The listing builds one solid part. Answer for the finished solid, in the listing's coordinates (mm). A direction names the side the tool comes from. Round coordinates to 2 decimals unless told otherwise and drop trailing zeros. Loops run counter-clockwise (first coordinate to the right, second up) from the corner with the lowest first, then second, coordinate; pieces in that order, holes last. Notation, with made-up numbers: M 34,69.25 L 93,69.25 A26 ccw 93,97.25 Z; hole C 59,-21 d3. An arc over 180 degrees is marked long. Answer as a JSON object with one key per item and string values.
```python
from build123d import *

# Parameters (mm, degrees)
BOSS_EXTRUDE1_DEPTH = 20
SKETCH2_W           = 5
SKETCH2_H           = 20
BOSS_EXTRUDE2_DEPTH = 5
CUT_EXTRUDE1_DEPTH  = 5
SKETCH4_W           = 5
SKETCH4_H           = 5
BOSS_EXTRUDE3_DEPTH = 5
CUT_EXTRUDE2_DEPTH  = 5
BOSS_EXTRUDE4_DEPTH = 20
CUT_EXTRUDE3_DEPTH  = 20
BOSS_EXTRUDE5_DEPTH = 5


with BuildPart() as part:
    # Sketch1 → Boss-Extrude1 (new body)
    with BuildSketch(Plane(origin=(0, 0, 0), x_dir=(1, 0, 0), z_dir=(0, 1, 0))):
        Polygon((-23.656387665, 13.90969163), (-8.656387665, 13.90969163), (-8.656387665, -1.09030837), (-18.656387665, 8.90969163), (-23.656387665, 8.90969163), align=None)
    extrude(amount=BOSS_EXTRUDE1_DEPTH)

    # Sketch2 → Boss-Extrude2 (add)
    with BuildSketch(Plane.ZY.offset(23.656387665)):
        with Locations((-11.40969163, 10)):
            Rectangle(SKETCH2_W, SKETCH2_H)
    extrude(amount=BOSS_EXTRUDE2_DEPTH)

    # Sketch3 → Cut-Extrude1 (cut)
    with BuildSketch(Plane.XY.offset(-8.90969163)):
        Polygon((-23.656387665, 20), (-28.656387665, 15), (-28.656387665, 20), align=None)
    extrude(amount=-CUT_EXTRUDE1_DEPTH, mode=Mode.SUBTRACT)

    # Sketch4 → Boss-Extrude3 (add)
    with BuildSketch(Plane.XY.offset(-8.90969163)):
        with Locations((-26.156387665, 2.5)):
            Rectangle(SKETCH4_W, SKETCH4_H)
    extrude(amount=BOSS_EXTRUDE3_DEPTH)

    # Sketch5 → Cut-Extrude2 (cut)
    with BuildSketch(Plane(origin=(0, 5, 0), x_dir=(1, 0, 0), z_dir=(0, 1, 0))):
        Polygon((-28.656387665, 8.90969163), (-23.656387665, 3.90969163), (-28.656387665, 3.90969163), align=None)
    extrude(amount=-CUT_EXTRUDE2_DEPTH, mode=Mode.SUBTRACT)

    # Sketch6 → Boss-Extrude4 (add)
    with BuildSketch(Plane(origin=(0, 0, 0), x_dir=(-1, 0, 0), z_dir=(0, -1, 0))):
        Polygon((18.656387665, -1.09030837), (23.656387665, 3.90969163), (23.656387665, 8.90969163), (18.656387665, 8.90969163), (8.656387665, -1.09030837), align=None)
    extrude(amount=-BOSS_EXTRUDE4_DEPTH)

    # 3DSketch1 → Cut-Extrude3 (cut, along a direction that is not the sketch's normal)
    with BuildSketch(Plane(origin=(-8.656387665, 20, 1.09030837), x_dir=(-0.8017837257372731, -0.26726124191242434, -0.5345224838248491), z_dir=(-0.577350269189626, 0.577350269189626, 0.5773502691896256))):
        Polygon((0, 0), (13.363062096, -4.629100499), (18.708286934, 0), (17.371980724, 6.943650748), (10.690449676, 9.258200998), align=None)
    extrude(amount=CUT_EXTRUDE3_DEPTH, dir=(0, 1, 0), mode=Mode.SUBTRACT)

    # Sketch7 → Boss-Extrude5 (add)
    with BuildSketch(Plane.XY.offset(1.09030837)):
        Polygon((-8.656387665, 15), (-13.656387665, 15), (-18.656387665, 10), (-18.656387665, 0), (-8.656387665, 0), align=None)
    extrude(amount=BOSS_EXTRUDE5_DEPTH)


solid = part.part
```
Item 1: The part is cut by section C-C (x = -17.25). Give the vertices of the cut face in (y, z), then the cut area to 3 significant figures.
Values follow:
{"outline": "M 0,-13.91 L 20,-13.91 L 20,-7.5 L 11.41,1.09 L 11.41,6.09 L 0,6.09 Z", "area": "320 mm^2"}
Item 2: Straight lines are drawn through the part: line 1 (Z direction, x = -25.5, y = 8.5); line 2 (X direction, y = 11, z = -5.5); line 3 (Y direction, x = -12.5, z = 3.75). For each, find the intervals that lie inside material, in ascending order.
Values follow:
{"line 1": "-13.91 to -8.91", "line 2": "-23.66 to -8.66", "line 3": "0 to 15"}
Item 3: Flat-ended cylindrical pins translate along their axes: P1, Ø4, axis at y = 9, z = -5.5, coming from the -X side; P2, Ø4, axis at y = 3, z = 2.5, coming from the -X side; P3, Ø1.5, axis at x = -20, y = 18.5, coming from the +Z side. Find the tip coordinate at first contact, or state that the pin passes through.
Values follow:
{"P1": "x = -23.66", "P2": "x = -19.25", "P3": "z = -7.69"}
Item 4: The part is cut by section B-B (z = 4.75). Give the vertices of the cut face in (x, y).
Values follow:
{"outline": "M -18.66,0 L -8.66,0 L -8.66,15 L -13.66,15 L -18.66,10 Z"}
Item 5: The part is cut by section A-A (y = 5.75). Give the vertices of the cut face in (x, z), then the cut area to 4 significant figures.
Values follow:
{"outline": "M -28.66,-13.91 L -8.66,-13.91 L -8.66,6.09 L -18.66,6.09 L -18.66,1.09 L -23.66,-3.91 L -23.66,-8.91 L -28.66,-8.91 Z", "area": "287.5 mm^2"}
Item 6: Which of the six approach directions +Z, -Z, +X, -X, +Y, -Y give full straight-line access (tool end or side, diameter ignored) to faces 1 (the face through (-11, 15, 4)), 2 (the face through (-23.656, 9, -6)), 3 (the face through (-18.656, 5, 4))?
Values follow:
{"face 1": "+Z, +X, -X, +Y", "face 2": "+Z, -X, +Y", "face 3": "+Z, -X, +Y, -Y"}
Item 7: The part is cut by section D-D (z = -7). Give the vertices of the cut face in (x, y).
Values follow:
{"outline": "M -26.75,0 L -8.66,0 L -8.66,20 L -16.75,20 L -23.66,13.09 L -23.66,5 L -26.75,5 Z"}
